Check sheet for the modelled part. Datum: model origin and axes. Units: mm. A direction names the side the tool comes from. Round coordinates to 2 decimals unless told otherwise and drop trailing zeros. Write each loop counter-clockwise with the first axis right and the second up, starting at its lowest first coordinate (ties: lowest second). Pieces come first, ordered by that corner, then holes.
from build123d import *

# Parameters (mm, degrees)
EXTRUDE_1_DEPTH    = 8
SKETCH1_R          = 1.6
CUT_EXTRUDE1_DEPTH = 2
SKETCH_2_R         = 1.6
CUT_EXTRUDE2_DEPTH = 16


with BuildPart() as part:
    # Эскиз1 → Бобышка-Вытянуть1 (new body)
    with BuildSketch(Plane.XY):
        Polygon((0, 0), (15, 0), (15, 1), (1, 1), (1, 15), (0, 15), align=None)
    extrude(amount=EXTRUDE_1_DEPTH)

    # Sketch1 → Cut-Extrude1 (cut, through all)
    with BuildSketch(Plane(origin=(1, 0, 0), x_dir=(0, 0, -1), z_dir=(1, 0, 0))):
        with Locations((-4, 10)):
            Circle(SKETCH1_R)
    extrude(amount=-CUT_EXTRUDE1_DEPTH, mode=Mode.SUBTRACT)

    # Эскиз2 → Cut-Extrude2 (cut, through all)
    with BuildSketch(Plane.XZ):
        with Locations((7.5, 4)):
            Circle(SKETCH_2_R)
    extrude(amount=-CUT_EXTRUDE2_DEPTH, mode=Mode.SUBTRACT)


solid = part.part
1. Sectioned sample at A-A, the plane y = 10. Enter the section's corners in (x, z).
2. Go/stop test with flat-tipped pins: pin 1 (4 mm diameter, centred on x = 11, z = 1.5, fed in from +Y); pin 2 (2.5 mm diameter, centred on y = 9, z = 5.5, fed in from +X). Record where each tip stops, or that it passes through.
3. Release check for a two-part mould opening along Y. For faces 3 (the flat face through (0.8, 4.2, 8)), 4 (the cylindrical face through (0.51, 8.44, 4.35)), 5 (the flat face through (10, 1, 4)) record: released by +Y, released by -Y, zero draft, split by the parting line, or undercut.
4. Sectioned sample at B-B, the plane z = 4. Enter the section's corners in (x, y).
5. Scan lines: line 1 along Y through (x, z) = (0.2, 4); line 2 along Z through (x, y) = (7.5, 0.55); line 3 along X through (y, z) = (4.5, 3). Record each from-to range of solid material in increasing order.
6. Set-up check for faces 1 (the flat face through (1, 8, 4)), 2 (the flat face through (0.8, 4.2, 0)): record each of +Z, -Z, +X, -X, +Y, -Y from which the full face is reachable in a straight line by a thin tool's end or side.
7. Sectioned sample at D-D, the plane z = 1.5. Enter the section's corners in (x, y).
Computed values:
1. outline: (0, 0) - (1, 0) - (1, 2.4) - (0, 2.4) - close; (0, 5.6) - (1, 5.6) - (1, 8) - (0, 8) - close
2. pin 1: stops at y = 1
2. pin 2: stops at x = 1
3. face 3: zero draft
3. face 4: undercut
3. face 5: released by +Y
4. outline: (0, 0) - (5.9, 0) - (5.9, 1) - (1, 1) - (1, 8.4) - (0, 8.4) - close; (0, 11.6) - (1, 11.6) - (1, 15) - (0, 15) - close; (9.1, 0) - (15, 0) - (15, 1) - (9.1, 1) - close
5. line 1: y = 0 to 8.4, 11.6 to 15
5. line 2: z = 0 to 2.4, 5.6 to 8
5. line 3: x = 0 to 1
6. face 1: +Z, -Z, +X, +Y
6. face 2: -Z, +X, -X, +Y, -Y
7. outline: (0, 0) - (15, 0) - (15, 1) - (1, 1) - (1, 15) - (0, 15) - close
